Autodesk Inventor part; units mm, degrees
ref_plane "YZ Plane" through (0, 0, 0) normal (1, 0, 0) x (0, 1, 0)
ref_plane "XZ Plane" through (0, 0, 0) normal (0, 1, 0) x (-1, 0, 0)
ref_plane "XY Plane" through (0, 0, 0) normal (0, 0, 1) x (1, 0, 0)
sketch "Skizze1" plane through (0, 0, 0) normal (0, 1, 0) x (-1, 0, 0)
  line L0 (0, -140) -> (0, 140)
  line L1 (-122.5, 0) -> (122.5, 0)
  line L2 (87.5, -100) -> (-87.5, -100)
  line L3 (-87.5, -100) -> (-87.5, 100)
  line L4 (-87.5, 100) -> (87.5, 100)
  line L5 (87.5, 100) -> (87.5, -100)
  point P0 (0, 0)
  dimension "d0" = 175
  dimension "d1" = 200
extrude "Extrusion1" add sketch "Skizze1" along normal blind 2
sketch "Skizze2" plane through (0, 2, 0) normal (0, 1, 0) x (1, 0, 0)
  circle A0 centre (70, 82.5) radius 1.6
  line L0 (87.5, -100) -> (87.5, 100)
  line L1 (87.5, 100) -> (-87.5, 100)
  circle A1 centre (70, 62.5) radius 1.6
  line L2 (122.5, 0) -> (-122.5, 0)
  circle A2 centre (70, -82.5) radius 1.6
  circle A3 centre (70, -62.5) radius 1.6
  point P0 (0, 0)
  dimension "d4" = 3.2
  dimension "d5" = 17.5
  dimension "d6" = 17.5
  dimension "d7" = 3.2
  dimension "d8" = 20
  dimension "d9" = 17.5
extrude "Extrusion2" cut sketch "Skizze2" against normal up to surface (2 mm away)
sketch "Skizze4" plane through (0, 2, 0) normal (0, 1, 0) x (1, 0, 0)
  line L0 (-87.5, -100) -> (87.5, -100)
  line L1 (-87.5, 100) -> (-87.5, -100)
  line L2 (87.5, -100) -> (-87.5, -100)
  line L3 (-87.5, -100) -> (-87.5, -98)
  line L4 (-87.5, -98) -> (87.5, -98)
  line L5 (87.5, -98) -> (87.5, -100)
  line L6 (87.5, 100) -> (-87.5, 100)
  line L7 (87.5, 100) -> (-87.5, 100)
  line L8 (-87.5, 100) -> (-87.5, 98)
  line L9 (-87.5, 98) -> (87.5, 98)
  line L10 (87.5, 98) -> (87.5, 100)
  line L11 (87.5, -98) -> (51.5, -98)
  line L12 (51.5, -98) -> (51.5, -92)
  line L13 (51.5, -92) -> (57.5, -92)
  line L14 (87.5, 98) -> (51.5, 98)
  line L15 (51.5, 98) -> (51.5, 92)
  line L16 (51.5, 92) -> (57.5, 92)
  line L17 (-87.5, -98) -> (-85.5, -98)
  line L18 (-85.5, -98) -> (-85.5, 98)
  line L19 (-85.5, 98) -> (-87.5, 98)
  line L20 (-87.5, 98) -> (-87.5, -98)
  line L21 (-85.5, 98) -> (-79.5, 98)
  line L22 (-79.5, 98) -> (-79.5, 92)
  line L23 (-79.5, 92) -> (-85.5, 92)
  line L24 (-85.5, 92) -> (-85.5, 98)
  line L25 (-85.5, -98) -> (-79.5, -98)
  line L26 (-79.5, -98) -> (-79.5, -92)
  line L27 (-79.5, -92) -> (-85.5, -92)
  line L28 (-85.5, -92) -> (-85.5, -98)
  line L29 (57.5, -92) -> (57.5, -98)
  line L30 (87.5, -100) -> (87.5, 100)
  line L31 (57.5, 98) -> (57.5, 92)
  point P0 (0, 0)
  point P1 (-85.5, -92)
  point P2 (51.5, -98)
  point P3 (-87.5, 98)
  point P4 (-87.5, 100)
  dimension "d18" = 2
  dimension "d19" = 2
  dimension "d21" = 6
  dimension "d23" = 6
  dimension "d24" = 2
  dimension "d25" = 6
  dimension "d26" = 6
  dimension "d27" = 6
  dimension "d28" = 6
  dimension "d130" = 6
  dimension "d131" = 30
  dimension "d132" = 6
  dimension "d133" = 30
extrude "Extrusion4" add sketch "Skizze4" along normal blind 50 contours L1 L4 L5 L0 | L1 L9 L18 L4 | L1 L6 L10 L9 | L18 L27 L26 L4 | L4 L12 L13 L29 | L9 L22 L23 L18 | L31 L16 L15 L9
sketch "Skizze5" plane through (0, 2, 0) normal (0, 1, 0) x (1, 0, 0)
  circle A0 centre (67.5, 35) radius 3.5
  circle A1 centre (67.5, -35) radius 3.5
  line L0 (-129.052, 0) -> (123.592, 0)
  line L1 (123.592, 0) -> (-129.052, 0)
  line L2 (87.5, -98) -> (87.5, 98)
  circle A2 centre (-5.5, -35) radius 3.5
  circle A3 centre (-5.5, 35) radius 3.5
  line L3 (87.5, 100) -> (-87.5, 100)
  circle A4 centre (-30, -48.325) radius 3.5
  circle A5 centre (-30, 34.225) radius 3.5
  circle A6 centre (-78.26, 27.875) radius 3.5
  circle A7 centre (-78.26, -47.055) radius 3.5
  line L4 (-87.5, 100) -> (-87.5, -100)
  line L5 (51.5, -98) -> (-79.5, -98)
  line L6 (-85.5, -92) -> (-85.5, 92)
  line L7 (0, 140) -> (0, -140)
  circle A8 centre (7.5, 49) radius 3.5
  circle A9 centre (7.5, 88) radius 3.5
  circle A10 centre (58.5, 49) radius 3.5
  circle A11 centre (58.5, 88) radius 3.5
  line L8 (-79.5, 98) -> (51.5, 98)
  circle A12 centre (7.5, -49) radius 3.5
  circle A13 centre (7.5, -88) radius 3.5
  circle A14 centre (58.5, -49) radius 3.5
  circle A15 centre (58.5, -88) radius 3.5
  circle A16 centre (-75.5, 56.5) radius 3.5
  circle A17 centre (-75.5, 90.5) radius 3.5
  circle A18 centre (-21.5, 56.5) radius 3.5
  circle A19 centre (-21.5, 90.5) radius 3.5
  circle A20 centre (-9, 73) radius 3.5
  circle A21 centre (-9, -73) radius 3.5
  point P0 (0, 0)
  point P1 (-75, 100)
  dimension "d31" = 7
  dimension "d32" = 7
  dimension "d35" = 20
  dimension "d36" = 20
  dimension "d37" = 7
  dimension "d38" = 73
  dimension "d40" = 7
  dimension "d42" = 73
  dimension "d68" = 70
  dimension "d69" = 70
  dimension "d70" = 35
  dimension "d73" = 65
  dimension "d74" = 7
  dimension "d75" = 7
  dimension "d83" = 7
  dimension "d86" = 7
  dimension "d136" = 48.26
  dimension "d137" = 74.93
  dimension "d138" = 48.26
  dimension "d139" = 82.55
  dimension "d142" = 30
  dimension "d143" = 30
  dimension "d144" = 34.225
  dimension "d145" = 47.055
  dimension "d148" = 7
  dimension "d149" = 7
  dimension "d150" = 7
  dimension "d151" = 7
  dimension "d152" = 10
  dimension "d153" = 10
  dimension "d154" = 39
  dimension "d155" = 39
  dimension "d156" = 51
  dimension "d157" = 51
  dimension "d161" = 7.5
  dimension "d163" = 7.5
  dimension "d177" = 7
  dimension "d178" = 7
  dimension "d179" = 7
  dimension "d180" = 7
  dimension "d181" = 10
  dimension "d182" = 10
  dimension "d183" = 7.5
  dimension "d184" = 34
  dimension "d185" = 7.5
  dimension "d186" = 34
  dimension "d187" = 54
  dimension "d188" = 54
  dimension "d193" = 7
  dimension "d194" = 25
  dimension "d195" = 9
  dimension "d196" = 7
  dimension "d197" = 25
  dimension "d198" = 9
extrude "Extrusion5" add sketch "Skizze5" along normal blind 7 contours A0 | A1 | A2 | A3 | A4 | A5 | A6 | A7 | A8 | A9 | A10 | A11 | A12 | A13 | A14 | A15 | A16 | A17 | A18 | A19 | A20 | A21
sketch "Skizze6" plane through (-5.5, 9, -35) normal (0, 1, 0) x (1, 0, 0)
  circle A0 centre (0, 0) radius 2
  circle A1 centre (73, 0) radius 3.5
  circle A2 centre (73, 0) radius 2
  circle A3 centre (0, -70) radius 2
  circle A4 centre (0, -70) radius 3.5
  circle A5 centre (73, -70) radius 3.5
  circle A6 centre (73, -70) radius 2
  circle A7 centre (-72.76, -82.055) radius 2
  circle A8 centre (-72.76, -82.055) radius 3.5
  circle A9 centre (-24.5, -83.325) radius 2
  circle A10 centre (-24.5, -83.325) radius 3.5
  circle A11 centre (-24.5, -0.775) radius 2
  circle A12 centre (-24.5, -0.775) radius 3.5
  circle A13 centre (-72.76, -7.125) radius 2
  circle A14 centre (-72.76, -7.125) radius 3.5
  circle A15 centre (13, -123) radius 3.5
  circle A16 centre (13, -123) radius 3.5
  circle A17 centre (13, -123) radius 2
  circle A18 centre (13, -84) radius 3.5
  circle A19 centre (13, -84) radius 3.5
  circle A20 centre (13, -84) radius 2
  circle A21 centre (64, -123) radius 2
  circle A22 centre (64, -123) radius 3.5
  circle A23 centre (64, -123) radius 3.5
  circle A24 centre (64, -84) radius 3.5
  circle A25 centre (64, -84) radius 3.5
  circle A26 centre (64, -84) radius 2
  line L0 (128, -35) -> (-117, -35)
  circle A27 centre (13, 53) radius 3.5
  circle A28 centre (13, 53) radius 2
  circle A29 centre (13, 14) radius 3.5
  circle A30 centre (13, 14) radius 2
  circle A31 centre (64, 53) radius 2
  circle A32 centre (64, 53) radius 3.5
  circle A33 centre (64, 14) radius 3.5
  circle A34 centre (64, 14) radius 2
  circle A35 centre (-70, 21.5) radius 3.5
  circle A36 centre (-70, 55.5) radius 3.5
  circle A37 centre (-16, 55.5) radius 3.5
  circle A38 centre (-16, 21.5) radius 3.5
  circle A39 centre (-70, 21.5) radius 2
  circle A40 centre (-70, 55.5) radius 3.5
  circle A41 centre (-70, 55.5) radius 2
  circle A42 centre (-16, 21.5) radius 3.5
  circle A43 centre (-16, 21.5) radius 2
  circle A44 centre (-16, 55.5) radius 3.5
  circle A45 centre (-16, 55.5) radius 2
  circle A46 centre (-3.5, -108) radius 3.5
  circle A47 centre (-3.5, 38) radius 3.5
  circle A48 centre (-3.5, -108) radius 2
  circle A49 centre (-3.5, 38) radius 3.5
  circle A50 centre (-3.5, 38) radius 2
  point P0 (-82, -78.8303)
  point P1 (-82, -84.6297)
  point P2 (-82, -3.9003)
  point P3 (-82, -9.6997)
  dimension "d45" = 4
  dimension "d46" = 4
  dimension "d47" = 4
  dimension "d48" = 0
  dimension "d49" = 4
  dimension "d50" = 73
  dimension "d51" = 70
  dimension "d96" = 4
  dimension "d97" = 0
  dimension "d98" = 0
  dimension "d99" = 4
  dimension "d100" = 0
  dimension "d101" = 0
  dimension "d102" = 4
  dimension "d103" = 0
  dimension "d104" = 4
  dimension "d105" = 0
  dimension "d164" = 7
  dimension "d165" = 0
  dimension "d166" = 0
  dimension "d167" = 4
  dimension "d168" = 7
  dimension "d169" = 0
  dimension "d170" = 4
  dimension "d171" = 4
  dimension "d172" = 0
  dimension "d173" = 7
  dimension "d174" = 7
  dimension "d176" = 4
  dimension "d189" = 4
  dimension "d190" = 4
  dimension "d191" = 4
  dimension "d192" = 4
  dimension "d199" = 4
  dimension "d200" = 4
extrude "Extrusion6" cut sketch "Skizze6" against normal blind 5 contours A0 | A2 | A3 | A6 | A7 | A9 | A11 | A13 | A17 | A20 | A21 | A26 | A28 | A30 | A31 | A34 | A39 | A41 | A43 | A45 | A48 | A50
sketch "Skizze7" plane through (0, 52, 0) normal (0, 1, 0) x (1, 0, 0)
  circle A0 centre (54.5, -95) radius 2
  circle A1 centre (-82.5, -95) radius 2
  circle A2 centre (-82.5, 95) radius 2
  circle A3 centre (54.5, 95) radius 2
  line L0 (51.5, 98) -> (51.5, 92)
  line L1 (51.5, 92) -> (57.5, 92)
  line L2 (51.5, -92) -> (51.5, -98)
  line L3 (57.5, -92) -> (51.5, -92)
  line L4 (-79.5, -98) -> (-79.5, -92)
  line L5 (-79.5, -92) -> (-85.5, -92)
  line L6 (-79.5, 92) -> (-79.5, 98)
  line L7 (-85.5, 92) -> (-79.5, 92)
  line L8 (57.5, -98) -> (57.5, -92)
  line L9 (57.5, 92) -> (57.5, 98)
  point P0 (0, 0)
  point P1 (75, -92)
  dimension "d54" = 4
  dimension "d55" = 4
  dimension "d56" = 4
  dimension "d57" = 4
  dimension "d59" = 3
  dimension "d61" = 3
  dimension "d62" = 3
  dimension "d63" = 3
  dimension "d64" = 3
  dimension "d65" = 3
  dimension "d146" = 3
  dimension "d147" = 3
extrude "Extrusion7" cut sketch "Skizze7" against normal blind 5
sketch "Skizze8" plane through (0, 2, 0) normal (0, 1, 0) x (1, 0, 0)
  circle A0 centre (69.5, 10) radius 1.6
  line L0 (122.5, 0) -> (-122.5, 0)
  line L1 (87.5, -98) -> (87.5, 98)
  circle A1 centre (69.5, -10) radius 1.6
  circle A2 centre (20.609, 42.961) radius 1.6
  circle A3 centre (17.873, 35.444) radius 1.6
  circle A4 centre (20.609, -42.961) radius 1.6
  circle A5 centre (17.873, -35.444) radius 1.6
  point P0 (0, 0)
  point P1 (75, -92)
  point P2 (75, 92)
  point P3 (87.5, 98)
  dimension "d119" = 3.2
  dimension "d120" = 18
  dimension "d121" = 10
  dimension "d122" = 3.2
  dimension "d123" = 3.2
  dimension "d124" = 66.891
  dimension "d125" = 69.627
  dimension "d126" = 42.961
  dimension "d127" = 35.444
extrude "Extrusion8" cut sketch "Skizze8" against normal up to surface (2 mm away)
equation "\"d43\" = d83"
properties part number "Grundplatte_vorne"
Can you work these out from the model? Positions are in its coordinate system, mm. A direction names the side the tool comes from. Give positions to 0.01 mm unless a question says otherwise; leave off trailing zeros. Order: outer loops, then holes, each group sorted by start corner. A loop starts at its lowest first (then second) coordinate and runs counter-clockwise, first axis right, second up. Notation, with made-up numbers: M -15.75,30 L -1.75,30 A22 cw -1.75,42 Z; hole C 31.25,10.25 d4. An arc over 180 degrees is marked long. Use a Markdown table: item, result. Add a question column.
Item 1: We'd pull the mould along Z, two halves only. Please class faces 1 (the flat face through (1, 26, 100)), 2 (the flat face through (-73, 9, -91)), 3 (the flat face through (-87.5, 26, 1)): +Z half, -Z half, draft (parallel to the pull), parting line (faces both ways), or undercut.
Item 2: Suppose I cut it at A-A (x = 76.5). List the corners of the cut face in (y, z) for me, then the cut area to 3 significant figures.
Item 3: If I drill on L1, parallel to X at y = 7, z = 88; L2, parallel to X at y = 0.5, z = 82.5; L3, parallel to Z at x = -46.5, y = 17.5, over which ranges is the centre line in solid material (lowest first)? Write a range as [from, to].
Item 4: For faces 4 (the flat face through (57.5, 27, -95)), 5 (the cylindrical face through (55.92, 5.451, -46.635)), which set-ups out of +Z, -Z, +X, -X, +Y, -Y let a thin tool reach every point of the face, with its end or its side?
Item 5: Suppose I cut it at C-C (y = 34). List the corners of the cut face in (x, z) for me, then the cut area to 3 significant figures.
Item 6: Suppose I cut it at B-B (z = 56). List the corners of the cut face in (x, y) for me.
Item 7: Will these pins go through, and if not, where does the flat tip stop? pin 1 (1.2 mm diameter, centred on x = 7.5, z = -87.5, fed in from +Y); pin 2 (3 mm diameter, centred on x = 59, z = 88.5, fed in from +Y); pin 3 (4 mm diameter, centred on y = 39.5, z = -73, fed in from +X).
Answer sheet:
| question | item | result |
|---|---|---|
| 1 | face 1 | +Z half |
| 1 | face 2 | undercut |
| 1 | face 3 | draft |
| 2 | outline | M 0,-100 L 52,-100 L 52,-98 L 2,-98 L 2,98 L 52,98 L 52,100 L 0,100 Z |
| 2 | area | 600 mm² |
| 3 | L1 | x = [-87.5, -85.5], [4, 5.5], [9.5, 11], [55, 56.5], [60.5, 62] |
| 3 | L2 | x = [-87.5, 68.4], [71.6, 87.5] |
| 3 | L3 | z = [-100, -98], [98, 100] |
| 4 | face 4 | +X, +Y |
| 4 | face 5 | +Y |
| 5 | outline | M -87.5,-100 L 87.5,-100 L 87.5,-98 L 57.5,-98 L 57.5,-92 L 51.5,-92 L 51.5,-98 L -79.5,-98 L -79.5,-92 L -85.5,-92 L -85.5,92 L -79.5,92 L -79.5,98 L 51.5,98 L 51.5,92 L 57.5,92 L 57.5,98 L 87.5,98 L 87.5,100 L -87.5,100 Z |
| 5 | area | 1,240 mm² |
| 6 | outline | M -87.5,0 L 87.5,0 L 87.5,2 L -85.5,2 L -85.5,52 L -87.5,52 Z |
| 7 | pin 1 | stops at y = 4 |
| 7 | pin 2 | stops at y = 9 |
| 7 | pin 3 | stops at x = -85.5 |
